Source: CAD feature listing. Evaluate the final solid. Frame: model axes, mm. A direction names the side the tool comes from. Round coordinates to 2 decimals unless told otherwise and drop trailing zeros. Write each loop counter-clockwise with the first axis right and the second up, starting at its lowest first coordinate (ties: lowest second). Pieces come first, ordered by that corner, then holes. Notation, with made-up numbers: M 14.25,-26 L 27.25,-26 A28 ccw 27.25,-1 Z; hole C -19,-29 d11. An arc over 180 degrees is marked long. Use a Markdown table: item, result.
```python
from build123d import *

# Parameters (mm, degrees)
SKETCH1_R           = 17
BOSS_EXTRUDE1_DEPTH = 1
SKETCH2_R           = 11
SKETCH2_R_2         = 9.652
BOSS_EXTRUDE2_DEPTH = 4


with BuildPart() as part:
    # Sketch1 → Boss-Extrude1 (new body)
    with BuildSketch(Plane(origin=(0, 0, 0), x_dir=(1, 0, 0), z_dir=(0, 1, 0))):
        with Locations(Location((0, 0, 0), (0, 0, 270))):
            Circle(SKETCH1_R)
    boss_extrude1 = extrude(amount=-BOSS_EXTRUDE1_DEPTH)

    # Sketch2 → Boss-Extrude2 (add)
    with BuildSketch(Plane(origin=(0, 0, 0), x_dir=(1, 0, 0), z_dir=(0, 1, 0))):
        with Locations(Location((0, 0, 0), (0, 0, 270))):
            Circle(SKETCH2_R)
        with Locations(Location((0, 0, 0), (0, 0, 270))):
            Circle(SKETCH2_R_2, mode=Mode.SUBTRACT)
    boss_extrude2 = extrude(amount=BOSS_EXTRUDE2_DEPTH)

    # Mirror1: Boss-Extrude1, Boss-Extrude2 across plane
    add(boss_extrude1.mirror(Plane.ZX.offset(-1)))
    add(boss_extrude2.mirror(Plane.ZX.offset(-1)))


solid = part.part
```
Q1. First-contact query: pin 1 Ø6 at (x, z) = (0, 3.5) entering from -Y; pin 2 Ø1 at (x, z) = (-7, -10.5) entering from +Y; pin 3 Ø3 at (y, z) = (-1, 5) entering from +X. Flat tips, straight axial feed; report the tip coordinate or a pass-through.
Results are:
| item | result |
|---|---|
| pin 1 | y = -2 |
| pin 2 | y = 0 |
| pin 3 | x = 16.64 |
Q2. Section A-A on z = 0. Return loops of the section in (x, y), plus the area to 3 significant figures.
Results are:
| item | result |
|---|---|
| outline | M -17,-2 L -11,-2 L -11,-6 L -9.65,-6 L -9.65,-2 L 9.65,-2 L 9.65,-6 L 11,-6 L 11,-2 L 17,-2 L 17,0 L 11,0 L 11,4 L 9.65,4 L 9.65,0 L -9.65,0 L -9.65,4 L -11,4 L -11,0 L -17,0 Z |
| area | 89.6 mm^2 |
Q3. Mould query, pull axis X, two halves, no side actions, for faces 1 (the cylindrical face through (-10.74, 1.97, -2.38)), 2 (the flat face through (-11, -2, 4)), 3 (the flat face through (0, -2, 0)). Classes: +X half, -X half, draft (parallel to the pull), parting line (faces both ways), or undercut.
Results are:
| item | result |
|---|---|
| face 1 | parting line |
| face 2 | draft |
| face 3 | undercut |
Q4. Section D-D on z = 12. Return loops of the section in (x, y), plus the area to 3 significant figures.
Results are:
| item | result |
|---|---|
| outline | M -12.04,-2 L 12.04,-2 L 12.04,0 L -12.04,0 Z |
| area | 48.2 mm^2 |
Q5. Reachability of faces 4 (the cylindrical face through (-5.87, -3.97, -7.66)), 5 (the flat face through (-11, 0, 4)), 6 (the cylindrical face through (16.855, -1.014, -2.213)) from +Z, -Z, +X, -X, +Y, -Y: full face, straight path, thin tool, end or side. Return the list, or none.
Results are:
| item | result |
|---|---|
| face 4 | -Y |
| face 5 | +Y |
| face 6 | +Y, -Y |
Q6. Line query: L1, parallel to X at y = -4.75, z = 0; L2, parallel to Y at x = -10, z = -9; L3, parallel to Z at x = 6, y = 3.5. Output: solid intervals per line, ascending.
Results are:
| item | result |
|---|---|
| L1 | -11 to -9.65, 9.65 to 11 |
| L2 | -2 to 0 |
| L3 | -9.22 to -7.56, 7.56 to 9.22 |
Q7. Section B-B on y = -2.75. Return loops of the section in (x, z).
Results are:
| item | result |
|---|---|
| outline | C 0,0 d22; hole C 0,0 d19.3 |
Q8. Section C-C on x = 6.5. Return loops of the section in (y, z).
Results are:
| item | result |
|---|---|
| outline | M -6,-8.87 L -2,-8.87 L -2,-15.71 L 0,-15.71 L 0,-8.87 L 4,-8.87 L 4,-7.14 L 0,-7.14 L 0,7.14 L 4,7.14 L 4,8.87 L 0,8.87 L 0,15.71 L -2,15.71 L -2,8.87 L -6,8.87 L -6,7.14 L -2,7.14 L -2,-7.14 L -6,-7.14 Z |
